Answer from the drawing. Dimensions are ordinates in mm from the lowest x, y and z of the part. A direction names the side the tool comes from. Round coordinates to 2 decimals unless told otherwise and drop trailing zeros. Write each loop counter-clockwise with the first axis right and the second up, starting at its lowest first coordinate (ties: lowest second). Pieces come first, ordered by that corner, then holes. Notation, with made-up numbers: (38, 16.25) - (43, 16.25) arc R28 ccw to (43, 43.25) - close; hole circle Ø7 at (59.25, -26.75). An arc over 180 degrees is marked (long way). Use a Markdown table: item, result. Add a question column.
1) A tool of negligible diameter and unlimited length cuts with its end or side. For the marked faces 5 and 6, from which of +Z, -Z, +X, -X, +Y, -Y can it reach the whole face along a straight path? Write none if from no direction.
2) A cutting plane is placed at C-C (y = 19). Give the vertices of the cut face in (x, z), then the cut area to 3 significant figures.
3) Determine the mould class of the marked faces 1, 2, 3 and 4 for opening direction Z: +Z half, -Z half, draft (parallel to the pull), parting line (faces both ways), or undercut.
4) A cutting plane is placed at B-B (x = 35). Give the vertices of the cut face in (y, z).
5) Each of these flat-tipped pins is pushed along its axis until it touches: P1, Ø5, axis at x = 79.98, z = 62.25, coming from the -Y side; P2, Ø3, axis at x = 31, z = 38.5, coming from the +Y side; P3, Ø6, axis at y = 9.5, z = 50, coming from the +X side. Where does it stop, or does it pass through?
6) A cutting plane is placed at A-A (z = 23.75). Give the vertices of the cut face in (x, y).
7) Find the intervals of material crossed by probe 1 along Z at (x, y) = (95, 39); probe 2 along X at (y, z) = (1.25, 15.6); probe 3 along X at (y, z) = (1.25, 23.75), in increasing order. Write a range as from..to.
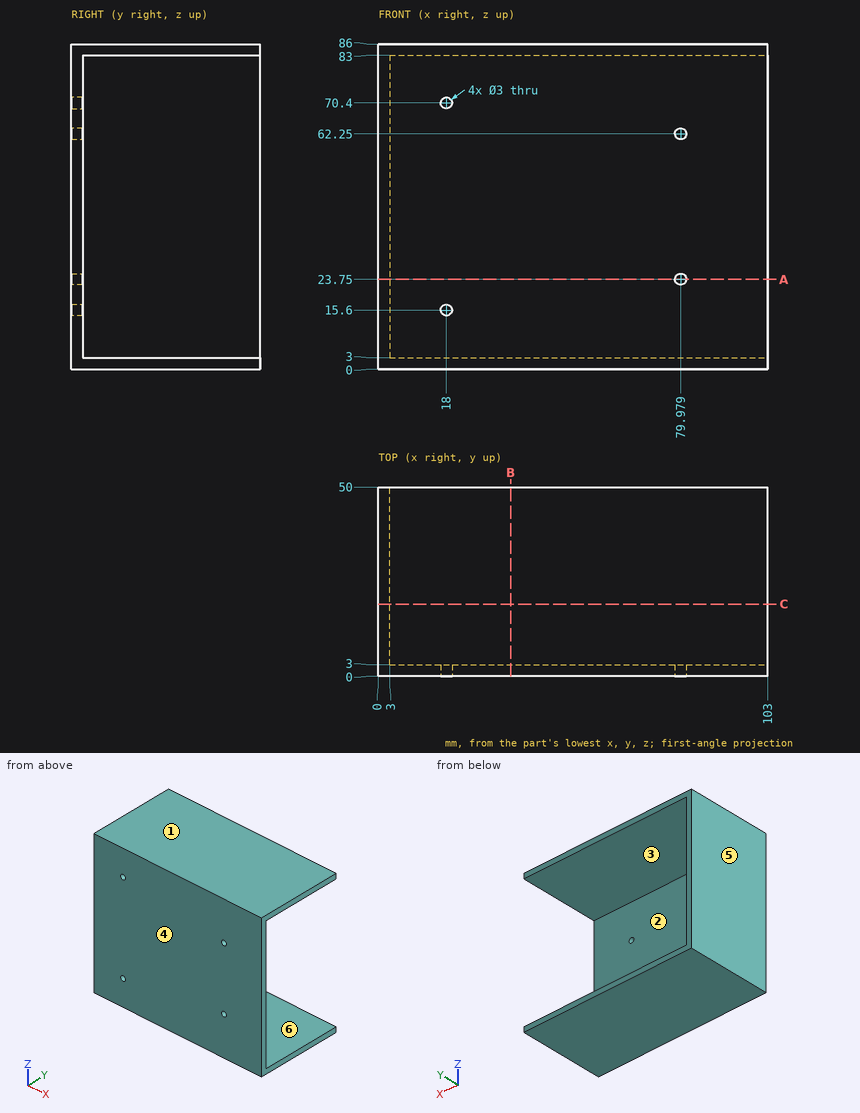
Entries:
| question | item | result |
|---|---|---|
| 1 | face 5 | +Z, -Z, -X, +Y, -Y |
| 1 | face 6 | +X, +Y |
| 2 | outline | (0, 0) - (103, 0) - (103, 3) - (3, 3) - (3, 83) - (103, 83) - (103, 86) - (0, 86) - close |
| 2 | area | 858 mm² |
| 3 | face 1 | +Z half |
| 3 | face 2 | undercut |
| 3 | face 3 | undercut |
| 3 | face 4 | draft |
| 4 | outline | (0, 0) - (50, 0) - (50, 3) - (3, 3) - (3, 83) - (50, 83) - (50, 86) - (0, 86) - close |
| 5 | P1 | stops at y = 0 |
| 5 | P2 | stops at y = 3 |
| 5 | P3 | stops at x = 3 |
| 6 | outline | (0, 0) - (78.48, 0) - (78.48, 3) - (3, 3) - (3, 50) - (0, 50) - close; (81.48, 0) - (103, 0) - (103, 3) - (81.48, 3) - close |
| 7 | probe 1 | z = 0..3, 83..86 |
| 7 | probe 2 | x = 0..16.5, 19.5..103 |
| 7 | probe 3 | x = 0..78.48, 81.48..103 |
